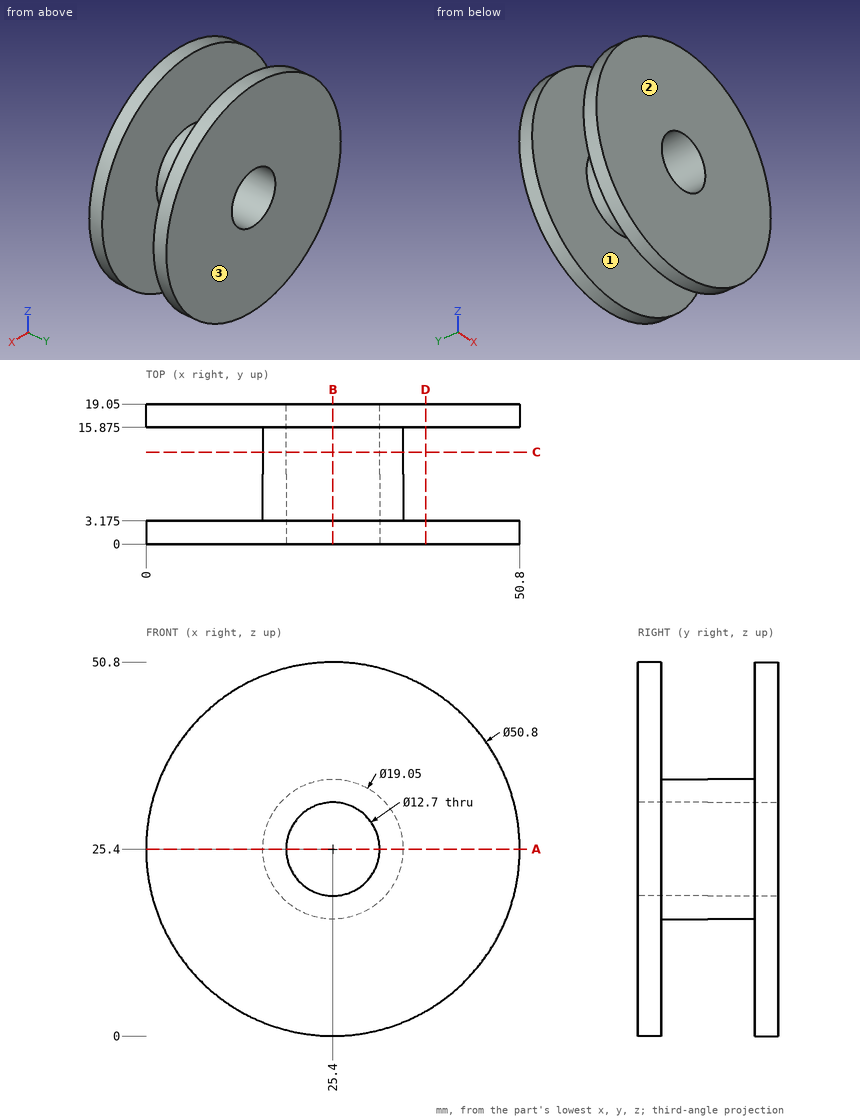
Study the drawing (mm; zero at the part's minimum x, y, z) and answer. Round coordinates to 2 decimals unless told otherwise and drop trailing zeros. Order: outer loops, then holes, each group sorted by start corner. A loop starts at its lowest first (then second) coordinate and runs counter-clockwise, first axis right, second up. Notation, with made-up numbers: (75, 23) - (96, 23) arc R10 ccw to (96, 38) - close; hole circle Ø7 at (25, 60.5). An arc over 180 degrees is marked (long way). Use one line per item in the form item = value. Start each with the question number.
(1) Flat-ended cylindrical pins translate along their axes: pin 1 Ø8 at (x, y) = (28, 14.5) entering from -Z; pin 2 Ø5 at (x, z) = (29, 6) entering from -Y; pin 3 Ø8 at (y, z) = (11.5, 6) entering from +X. Find the tip coordinate at first contact, or state that the pin passes through.
(2) The part is cut by section C-C (y = 12.5). Give the vertices of the cut face in (x, z) (3 decimals), then the cut area to 3 significant figures.
(3) Find the intervals of material crossed by line 1 along Y through (x, z) = (25, 15) (3 decimals); line 2 along Z through (x, y) = (25.4, 7.25) (3 decimals), in increasing order. Write a range as from..to.
(4) The part is cut by section D-D (x = 38). Give the vertices of the cut face in (y, z) (3 decimals), then the cut area to 3 significant figures.
(5) The part is cut by section A-A (z = 25.4). Give the vertices of the cut face in (x, y) (3 decimals), then the cut area to 3 significant figures.
(6) The part is cut by section B-B (x = 25.4). Give the vertices of the cut face in (y, z) (3 decimals), then the cut area to 3 significant figures.
(7) Determine the mould class of the marked faces 1, 2 and 3 for opening direction Y: +Y half, -Y half, draft (parallel to the pull), parting line (faces both ways), or undercut.
Checked values:
q1.pin_1 = 0
q1.pin_2 = 0
q1.pin_3 = through
q2.outline = circle Ø19.05 at (25.4, 25.4); hole circle Ø12.7 at (25.4, 25.4)
q2.area = 158 mm^2
q3.line_1 = 0..3.175, 15.875..19.05
q3.line_2 = 15.875..19.05, 31.75..34.925
q4.outline = (0, 3.346) - (3.175, 3.346) - (3.175, 47.454) - (0, 47.454) - close; (15.875, 3.346) - (19.05, 3.346) - (19.05, 47.454) - (15.875, 47.454) - close
q4.area = 280 mm^2
q5.outline = (0, 0) - (19.05, 0) - (19.05, 19.05) - (0, 19.05) - (0, 15.875) - (15.875, 15.875) - (15.875, 3.175) - (0, 3.175) - close; (31.75, 0) - (50.8, 0) - (50.8, 3.175) - (34.925, 3.175) - (34.925, 15.875) - (50.8, 15.875) - (50.8, 19.05) - (31.75, 19.05) - close
q5.area = 323 mm^2
q6.outline = (0, 0) - (3.175, 0) - (3.175, 15.875) - (15.875, 15.875) - (15.875, 0) - (19.05, 0) - (19.05, 19.05) - (0, 19.05) - close; (0, 31.75) - (19.05, 31.75) - (19.05, 50.8) - (15.875, 50.8) - (15.875, 34.925) - (3.175, 34.925) - (3.175, 50.8) - (0, 50.8) - close
q6.area = 323 mm^2
q7.face_1 = undercut
q7.face_2 = -Y half
q7.face_3 = +Y half
